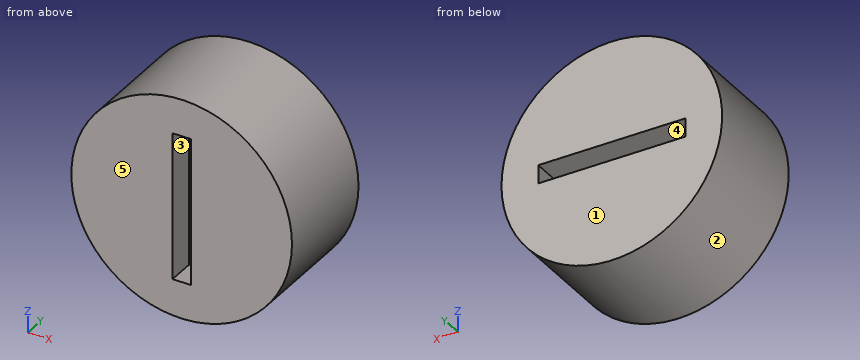
```python
from build123d import *

# Parameters (mm, degrees)
SKIZZE1_R                       = 6
AUFSATZ_LINEAR_AUSTRAGEN1_DEPTH = 6
SKIZZE2_W                       = 8
SKIZZE2_H                       = 1
SCHNITT_LINEAR_AUSTRAGEN1_DEPTH = 1.5
SKIZZE3_W                       = 1
SKIZZE3_H                       = 8
SCHNITT_LINEAR_AUSTRAGEN2_DEPTH = 1.5


with BuildPart() as part:
    # Skizze1 → Aufsatz-Linear austragen1 (new body)
    with BuildSketch(Plane(origin=(0, 0, 0), x_dir=(1, 0, 0), z_dir=(0, 1, 0))):
        Circle(SKIZZE1_R)
    extrude(amount=AUFSATZ_LINEAR_AUSTRAGEN1_DEPTH)

    # Skizze2 → Schnitt-Linear austragen1 (cut)
    with BuildSketch(Plane(origin=(0, 6, 0), x_dir=(1, 0, 0), z_dir=(0, 1, 0))):
        Rectangle(SKIZZE2_W, SKIZZE2_H)
    extrude(amount=-SCHNITT_LINEAR_AUSTRAGEN1_DEPTH, mode=Mode.SUBTRACT)

    # Skizze3 → Schnitt-Linear austragen2 (cut)
    with BuildSketch(Plane.XZ):
        Rectangle(SKIZZE3_W, SKIZZE3_H)
    extrude(amount=-SCHNITT_LINEAR_AUSTRAGEN2_DEPTH, mode=Mode.SUBTRACT)


solid = part.part
```
Could you check a few things on this model? Use its own coordinates, in mm. Face numbers are marked on the shaded views. A direction names the side the tool comes from. Round coordinates to 2 decimals unless told otherwise and drop trailing zeros. Loops run counter-clockwise (first coordinate to the right, second up) from the corner with the lowest first, then second, coordinate; pieces in that order, holes last. Notation, with made-up numbers: (60.25, 53) - (106.25, 53) arc R36 ccw to (106.25, 91) - close; hole circle Ø1 at (16.25, -23). An arc over 180 degrees is marked (long way). Use CSV: the item, a comma, the result in double quotes.
Item 1: If we mould it in two halves opening along Z, with no side actions, what happens to the marked faces 1, 2 and 3? For each: pulls with the +Z half, pulls with the -Z half, needs draft (parallel to the pull), parting line crosses it, or undercut.
Here are the results:
face 1,"needs draft"
face 2,"parting line crosses it"
face 3,"undercut"
Item 2: If we section it at D-D on y = 1.8: List the corners of the cut face in (x, z) for me, then the cut area to 3 significant figures.
Here are the results:
outline,"circle Ø12 at (0, 0)"
area,"113 mm²"
Item 3: If we section it at C-C on y = 0.7: List the corners of the cut face in (x, z) for me, then the cut area to 3 significant figures.
Here are the results:
outline,"circle Ø12 at (0, 0); hole (-0.5, -4) - (0.5, -4) - (0.5, 4) - (-0.5, 4) - close"
area,"105 mm²"
Item 4: For the marked faces 4 and 5, which set-ups out of +Z, -Z, +X, -X, +Y, -Y let a thin tool reach every point of the face, with its end or its side?
Here are the results:
face 4,"+Y"
face 5,"+Z, -Z, +X, -X, -Y"
Item 5: If we section it at A-A on x = 0: List the corners of the cut face in (y, z) for me.
Here are the results:
outline,"(0, -6) - (6, -6) - (6, -0.5) - (4.5, -0.5) - (4.5, 0.5) - (6, 0.5) - (6, 6) - (0, 6) - (0, 4) - (1.5, 4) - (1.5, -4) - (0, -4) - close"
Item 6: If we section it at B-B on z = 0: List the corners of the cut face in (x, y) for me.
Here are the results:
outline,"(-6, 0) - (-0.5, 0) - (-0.5, 1.5) - (0.5, 1.5) - (0.5, 0) - (6, 0) - (6, 6) - (4, 6) - (4, 4.5) - (-4, 4.5) - (-4, 6) - (-6, 6) - close"
Item 7: I need wall thicknesses on L1, parallel to Z at x = 0, y = 5.4; L2, parallel to Z at x = 1, y = 5.05; L3, parallel to Z at x = -1.75, y = 3.75. Which ranges of each line are inside material? Lowest first, please. Write a range as [from, to].
Here are the results:
L1,"z = [-6, -0.5], [0.5, 6]"
L2,"z = [-5.92, -0.5], [0.5, 5.92]"
L3,"z = [-5.74, 5.74]"
Item 8: Will these pins go through, and if not, where does the flat tip stop? pin 1 (0.5 mm diameter, centred on x = 0, z = -0.5, fed in from -Y); pin 2 (3 mm diameter, centred on y = 5.5, z = -3.5, fed in from -X); pin 3 (2 mm diameter, centred on y = 2.5, z = -4.5, fed in from -X).
Here are the results:
pin 1,"stops at y = 1.5"
pin 2,"stops at x = -5.66"
pin 3,"stops at x = -4.87"
